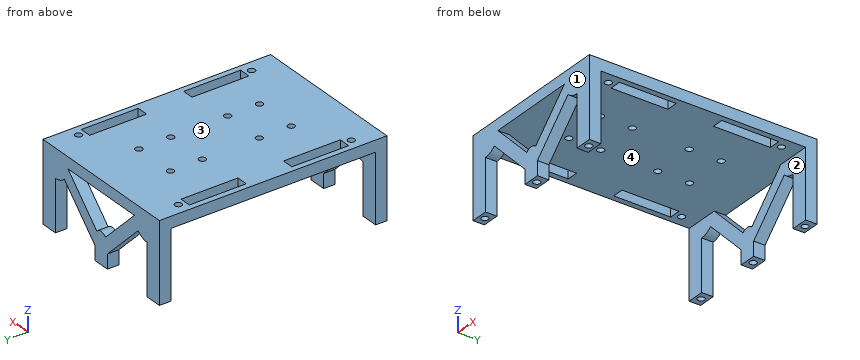
from build123d import *

# Parameters (mm, degrees)
SKETCH1_W           = 70
SKETCH1_H           = 100
BOSS_EXTRUDE1_DEPTH = 2.5
SKETCH2_R           = 1.5
CUT_EXTRUDE1_DEPTH  = 10
BOSS_EXTRUDE2_DEPTH = 5
SKETCH4_W           = 5
SKETCH4_H           = 25
SKETCH4_R           = 1.5
CUT_EXTRUDE2_DEPTH  = 5
SKETCH7_R           = 1.5
CUT_EXTRUDE3_DEPTH  = 5


with BuildPart() as part:
    # Sketch1 → Boss-Extrude1 (new, symmetric)
    with BuildSketch(Plane.XY):
        Rectangle(SKETCH1_W, SKETCH1_H)
    extrude(amount=BOSS_EXTRUDE1_DEPTH, both=True)

    # Sketch2 → Cut-Extrude1 (cut)
    with BuildSketch(Plane(origin=(0, 0, -2.5), x_dir=(-1, 0, 0), z_dir=(0, 0, -1))):
        with Locations((30, 38)):
            Circle(SKETCH2_R)
        with Locations((-30, 38)):
            Circle(SKETCH2_R)
        with Locations((30, -38)):
            Circle(SKETCH2_R)
        with Locations((-30, -38)):
            Circle(SKETCH2_R)
    extrude(amount=-CUT_EXTRUDE1_DEPTH, mode=Mode.SUBTRACT)

    # Sketch3 → Boss-Extrude2 (add)
    with BuildSketch(Plane(origin=(0, 50, 0), x_dir=(1, 0, 0), z_dir=(0, 1, 0))):
        with BuildLine():
            Line((-35, 2.5), (-35, 32.5))
            Line((-35, 32.5), (-27.5, 32.5))
            Line((-27.5, 32.5), (-27.5, 10))
            ThreePointArc((-27.5, 10), (-24.629874257, 9.429096494), (-22.196699141, 7.803300859))
            Line((-22.196699141, 7.803300859), (-3.75, 26.25))
            Line((-3.75, 26.25), (-3.75, 32.5))
            Line((-3.75, 32.5), (3.75, 32.5))
            Line((3.75, 32.5), (3.75, 26.25))
            Line((3.75, 26.25), (22.196699141, 7.803300859))
            ThreePointArc((22.196699141, 7.803300859), (24.629874257, 9.429096494), (27.5, 10))
            Line((27.5, 10), (27.5, 32.5))
            Line((27.5, 32.5), (35, 32.5))
            Line((35, 32.5), (35, 2.5))
            Line((35, 2.5), (20, 2.5))
            Line((20, 2.5), (2.651650429, 19.848349571))
            ThreePointArc((2.651650429, 19.848349571), (0, 18.75), (-2.651650429, 19.848349571))
            Line((-2.651650429, 19.848349571), (-20, 2.5))
            Line((-20, 2.5), (-35, 2.5))
        make_face()
    boss_extrude2 = extrude(amount=-BOSS_EXTRUDE2_DEPTH)

    # Mirror1: Boss-Extrude2 across plane
    add(boss_extrude2.mirror(Plane.ZX))

    # Sketch4 → Cut-Extrude2 (cut)
    with BuildSketch(Plane(origin=(0, 0, -2.5), x_dir=(-1, 0, 0), z_dir=(0, 0, -1))):
        with Locations((-30, -22.5)):
            Rectangle(SKETCH4_W, SKETCH4_H)
        with Locations(Location((-9.5, -26.5, 0), (0, 0, 180))):
            Circle(SKETCH4_R)
        with Locations(Location((-9.5, -12.5, 0), (0, 0, 180))):
            Circle(SKETCH4_R)
        with Locations((9.5, -12.5)):
            Circle(SKETCH4_R)
        with Locations((9.5, -26.5)):
            Circle(SKETCH4_R)
        with Locations((30, -22.5)):
            Rectangle(SKETCH4_W, SKETCH4_H)
        with Locations((30, 22.5)):
            Rectangle(SKETCH4_W, SKETCH4_H)
        with Locations(Location((9.5, 12.5, 0), (0, 0, 180))):
            Circle(SKETCH4_R)
        with Locations(Location((9.5, 26.5, 0), (0, 0, 180))):
            Circle(SKETCH4_R)
        with Locations((-9.5, 26.5)):
            Circle(SKETCH4_R)
        with Locations((-9.5, 12.5)):
            Circle(SKETCH4_R)
        with Locations((-30, 22.5)):
            Rectangle(SKETCH4_W, SKETCH4_H)
    extrude(amount=-CUT_EXTRUDE2_DEPTH, mode=Mode.SUBTRACT)

    # Sketch7 → Cut-Extrude3 (cut)
    with BuildSketch(Plane(origin=(0, 0, -32.5), x_dir=(-1, 0, 0), z_dir=(0, 0, -1))):
        with Locations((0, 47.5)):
            Circle(SKETCH7_R)
        with Locations((-31.25, 47.5)):
            Circle(SKETCH7_R)
        with Locations((31.25, 47.5)):
            Circle(SKETCH7_R)
    cut_extrude3 = extrude(amount=-CUT_EXTRUDE3_DEPTH, mode=Mode.SUBTRACT)

    # Mirror2: Cut-Extrude3 across plane
    add(cut_extrude3.mirror(Plane.ZX), mode=Mode.SUBTRACT)


solid = part.part
Input: part model. Units: mm. Frame: model coordinates. Face numbers are marked on the shaded views. Round coordinates to 2 decimals unless told otherwise and drop trailing zeros. Write each loop counter-clockwise with the first axis right and the second up, starting at its lowest first coordinate (ties: lowest second). Pieces come first, ordered by that corner, then holes.
1) Cut plane A-A (z = -29). Count the separate pieces of the cut face and the enclosed holes in it, then the cut area to 3 significant figures.
2) Cut plane C-C (x = 0). Return the cut outline in (y, z).
3) Draft query along Y for the marked faces 1, 2, 3 and 4. Return one class per face: pulls with the +Y half, pulls with the -Y half, needs draft (parallel to the pull), parting line crosses it, or undercut.
4) Ray query, L1, parallel to Y at x = 30, z = -0.45; L2, parallel to Y at x = -9.5, z = -0.65; L3, parallel to X at y = 47, z = -30. Return the intervals inside material, ascending.
5) Cut plane B-B (y = 12.5). Return the cut outline in (x, z), then the cut area to 3 significant figures.
6) Contact query for a flat-ended pin moving along its axis: P1, Ø4, axis at x = -7, y = 30.5, coming from the -Z side. Output: stop coordinate, or through.
Geometry says:
1. separate pieces: 6
1. enclosed holes: 6
1. area: 183 mm2
2. outline: (-50, -32.5) - (-49, -32.5) - (-49, -27.5) - (-46, -27.5) - (-46, -32.5) - (-45, -32.5) - (-45, -18.75) - (-50, -18.75) - close; (-50, -2.5) - (50, -2.5) - (50, 2.5) - (-50, 2.5) - close; (45, -32.5) - (46, -32.5) - (46, -27.5) - (49, -27.5) - (49, -32.5) - (50, -32.5) - (50, -18.75) - (45, -18.75) - close
3. face 1: pulls with the -Y half
3. face 2: undercut
3. face 3: needs draft
3. face 4: undercut
4. L1: y = -50 to -39.5, -36.5 to -35, -10 to 10, 35 to 36.5, 39.5 to 50
4. L2: y = -50 to -28, -25 to -14, -11 to 11, 14 to 25, 28 to 50
4. L3: x = -35 to -32.66, -29.84 to -27.5, -3.75 to -1.41, 1.41 to 3.75, 27.5 to 29.84, 32.66 to 35
5. outline: (-35, -2.5) - (-32.5, -2.5) - (-32.5, 2.5) - (-35, 2.5) - close; (-27.5, -2.5) - (-11, -2.5) - (-11, 2.5) - (-27.5, 2.5) - close; (-8, -2.5) - (8, -2.5) - (8, 2.5) - (-8, 2.5) - close; (11, -2.5) - (27.5, -2.5) - (27.5, 2.5) - (11, 2.5) - close; (32.5, -2.5) - (35, -2.5) - (35, 2.5) - (32.5, 2.5) - close
5. area: 270 mm2
6. P1: stops at z = -2.5
